```python
from build123d import *

# Parameters (mm, degrees)
BOSS_EXTRUDE1_DEPTH = 100
SKETCH2_R           = 10
CUT_EXTRUDE1_DEPTH  = 140.26


with BuildPart() as part:
    # Sketch1 → Boss-Extrude1 (new body)
    with BuildSketch(Plane.XY):
        with BuildLine():
            Line((-23.336691171, 0), (20.163308829, 0))
            ThreePointArc((20.163308829, 0), (27.234376641, 2.928932188), (30.163308829, 10))
            Line((30.163308829, 10), (30.163308829, 53.5))
            ThreePointArc((30.163308829, 53.5), (33.092241017, 60.571067812), (40.163308829, 63.5))
            Line((40.163308829, 63.5), (80.163308829, 63.5))
            Line((80.163308829, 63.5), (120.163308829, 63.5))
            ThreePointArc((120.163308829, 63.5), (127.234376641, 60.571067812), (130.163308829, 53.5))
            Line((130.163308829, 53.5), (130.163308829, 10))
            ThreePointArc((130.163308829, 10), (133.092241017, 2.928932188), (140.163308829, 0))
            Line((140.163308829, 0), (183.663308829, 0))
            ThreePointArc((183.663308829, 0), (190.734376641, 2.928932188), (193.663308829, 10))
            Line((193.663308829, 10), (193.663308829, 53.5))
            ThreePointArc((193.663308829, 53.5), (196.592241017, 60.571067812), (203.663308829, 63.5))
            Line((203.663308829, 63.5), (293.663308829, 63.5))
            Line((293.663308829, 63.5), (293.663308829, 50.8))
            Line((293.663308829, 50.8), (216.363308829, 50.8))
            ThreePointArc((216.363308829, 50.8), (209.292241017, 47.871067812), (206.363308829, 40.8))
            Line((206.363308829, 40.8), (206.363308829, -2.7))
            ThreePointArc((206.363308829, -2.7), (203.434376641, -9.771067812), (196.363308829, -12.7))
            Line((196.363308829, -12.7), (127.463308829, -12.7))
            ThreePointArc((127.463308829, -12.7), (120.392241017, -9.771067812), (117.463308829, -2.7))
            Line((117.463308829, -2.7), (117.463308829, 40.8))
            ThreePointArc((117.463308829, 40.8), (114.534376641, 47.871067812), (107.463308829, 50.8))
            Line((107.463308829, 50.8), (80.163308829, 50.8))
            Line((80.163308829, 50.8), (52.863308829, 50.8))
            ThreePointArc((52.863308829, 50.8), (45.792241017, 47.871067812), (42.863308829, 40.8))
            Line((42.863308829, 40.8), (42.863308829, -2.7))
            ThreePointArc((42.863308829, -2.7), (39.934376641, -9.771067812), (32.863308829, -12.7))
            Line((32.863308829, -12.7), (-36.036691171, -12.7))
            ThreePointArc((-36.036691171, -12.7), (-43.107758983, -9.771067812), (-46.036691171, -2.7))
            Line((-46.036691171, -2.7), (-46.036691171, 40.8))
            ThreePointArc((-46.036691171, 40.8), (-48.965623359, 47.871067812), (-56.036691171, 50.8))
            Line((-56.036691171, 50.8), (-83.336691171, 50.8))
            Line((-83.336691171, 50.8), (-110.636691171, 50.8))
            ThreePointArc((-110.636691171, 50.8), (-117.707758983, 47.871067812), (-120.636691171, 40.8))
            Line((-120.636691171, 40.8), (-120.636691171, -2.7))
            ThreePointArc((-120.636691171, -2.7), (-123.565623359, -9.771067812), (-130.636691171, -12.7))
            Line((-130.636691171, -12.7), (-199.536691171, -12.7))
            ThreePointArc((-199.536691171, -12.7), (-206.607758983, -9.771067812), (-209.536691171, -2.7))
            Line((-209.536691171, -2.7), (-209.536691171, 40.8))
            ThreePointArc((-209.536691171, 40.8), (-212.465623359, 47.871067812), (-219.536691171, 50.8))
            Line((-219.536691171, 50.8), (-296.836691171, 50.8))
            Line((-296.836691171, 50.8), (-296.836691171, 63.5))
            Line((-296.836691171, 63.5), (-206.836691171, 63.5))
            ThreePointArc((-206.836691171, 63.5), (-199.765623359, 60.571067812), (-196.836691171, 53.5))
            Line((-196.836691171, 53.5), (-196.836691171, 10))
            ThreePointArc((-196.836691171, 10), (-193.907758983, 2.928932188), (-186.836691171, 0))
            Line((-186.836691171, 0), (-143.336691171, 0))
            ThreePointArc((-143.336691171, 0), (-136.265623359, 2.928932188), (-133.336691171, 10))
            Line((-133.336691171, 10), (-133.336691171, 53.5))
            ThreePointArc((-133.336691171, 53.5), (-130.407758983, 60.571067812), (-123.336691171, 63.5))
            Line((-123.336691171, 63.5), (-83.336691171, 63.5))
            Line((-83.336691171, 63.5), (-43.336691171, 63.5))
            ThreePointArc((-43.336691171, 63.5), (-36.265623359, 60.571067812), (-33.336691171, 53.5))
            Line((-33.336691171, 53.5), (-33.336691171, 10))
            ThreePointArc((-33.336691171, 10), (-30.407758983, 2.928932188), (-23.336691171, 0))
        make_face()
    extrude(amount=BOSS_EXTRUDE1_DEPTH)

    # Sketch2 → Cut-Extrude1 (cut)
    with BuildSketch(Plane(origin=(0, 0, 0), x_dir=(1, 0, 0), z_dir=(0, 1, 0))):
        with Locations((-258.186691171, -75)):
            Circle(SKETCH2_R)
        with Locations((-258.186691171, -25)):
            Circle(SKETCH2_R)
        with Locations(Location((-83.336691171, -75, 0), (0, 0, 180))):
            Circle(SKETCH2_R)
        with Locations(Location((-83.336691171, -25, 0), (0, 0, 180))):
            Circle(SKETCH2_R)
        with Locations(Location((80.163308829, -75, 0), (0, 0, 90))):
            Circle(SKETCH2_R)
        with Locations(Location((80.163308829, -25, 0), (0, 0, 90))):
            Circle(SKETCH2_R)
        with Locations((255.013308829, -75)):
            Circle(SKETCH2_R)
        with Locations((255.013308829, -25)):
            Circle(SKETCH2_R)
    extrude(amount=CUT_EXTRUDE1_DEPTH, mode=Mode.SUBTRACT)


solid = part.part
```
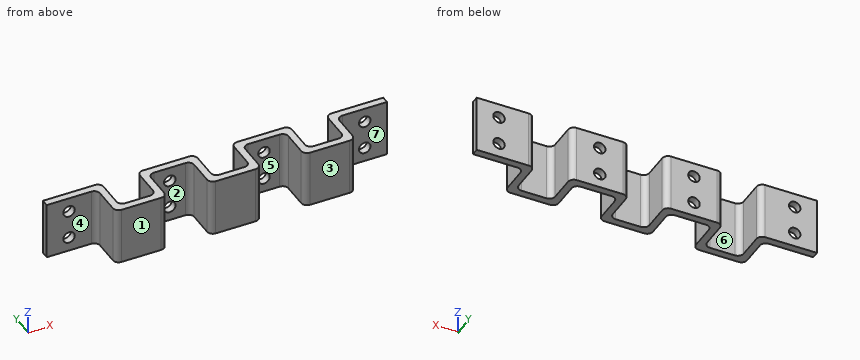
Verification items for the finished model (mm, model axes). Face numbers are marked on the shaded views. A direction names the side the tool comes from. Round coordinates to 2 decimals unless told otherwise and drop trailing zeros. Order: outer loops, then holes, each group sorted by start corner. A loop starts at its lowest first (then second) coordinate and runs counter-clockwise, first axis right, second up. Notation, with made-up numbers: (-35, 81) - (13, 81) arc R30 ccw to (13, 103) - close; hole circle Ø5 at (-27, 1.25). An arc over 180 degrees is marked (long way). Use CSV: the item, a comma, the result in double quotes.
(1) Gauge pin test, flat ends, axial feed: pin 1 Ø2 at (y, z) = (44, 58.5) entering from +X; pin 2 Ø13 at (y, z) = (34, 65) entering from -X; pin 3 Ø22 at (y, z) = (33, 45.5) entering from +X; pin 4 Ø16 at (x, z) = (80.16, 25) entering from +Y. Record the tip position at first contact, or that the pin passes through.
Entries:
pin 1,"x = 207.29"
pin 2,"x = -209.54"
pin 3,"x = 206.89"
pin 4,"through"
(2) Mould release check, pull along X, two halves, no side actions. Record for the marked faces 1 and 2: released by +X, released by -X, zero draft, split by the parting line, or undercut.
Entries:
face 1,"zero draft"
face 2,"undercut"
(3) Thickness scan on probe 1 along X at (y, z) = (25, 24.5); probe 2 along X at (y, z) = (-3.5, 34.5); probe 3 along X at (y, z) = (42.5, 32.5). Record the ranges inside material, lowest first. Write a range as from..to.
Entries:
probe 1,"-209.54..-196.84, -133.34..-120.64, -46.04..-33.34, 30.16..42.86, 117.46..130.16, 193.66..206.36"
probe 2,"-209.5..-120.67, -46..42.83, 117.5..206.33"
probe 3,"-209.68..-196.84, -133.34..-120.49, -46.18..-33.34, 30.16..43.01, 117.32..130.16, 193.66..206.51"
(4) Section check C-C on x = 164.5. Record the boundary of the cut face in (y, z), and give its area (3 significant figures).
Entries:
outline,"(-12.7, 0) - (0, 0) - (0, 100) - (-12.7, 100) - close"
area,"1,270 mm^2"
(5) Access from +Z, -Z, +X, -X, +Y, -Y to the whole of each face (thin tool, end or side, straight path). Record for the marked faces 3, 4, 5, 6 and 7.
Entries:
face 3,"+Z, -Z, +X, -X, -Y"
face 4,"+Z, -Z, -X, -Y"
face 5,"+Z, -Z, -Y"
face 6,"+Z, -Z, +Y"
face 7,"+Z, -Z, +X, -Y"
(6) Section check B-B on z = 25. State how many separate pieces and enclosed holes the cut face has, and give its area (3 significant figures).
Entries:
separate pieces,"5"
enclosed holes,"0"
area,"11,300 mm^2"
(7) Section check A-A on y = 20. Record the boundary of the cut face in (x, z), and give its area (3 significant figures).
Entries:
outline,"(-209.54, 0) - (-196.84, 0) - (-196.84, 100) - (-209.54, 100) - close; (-133.34, 0) - (-120.64, 0) - (-120.64, 100) - (-133.34, 100) - close; (-46.04, 0) - (-33.34, 0) - (-33.34, 100) - (-46.04, 100) - close; (30.16, 0) - (42.86, 0) - (42.86, 100) - (30.16, 100) - close; (117.46, 0) - (130.16, 0) - (130.16, 100) - (117.46, 100) - close; (193.66, 0) - (206.36, 0) - (206.36, 100) - (193.66, 100) - close"
area,"7,620 mm^2"
